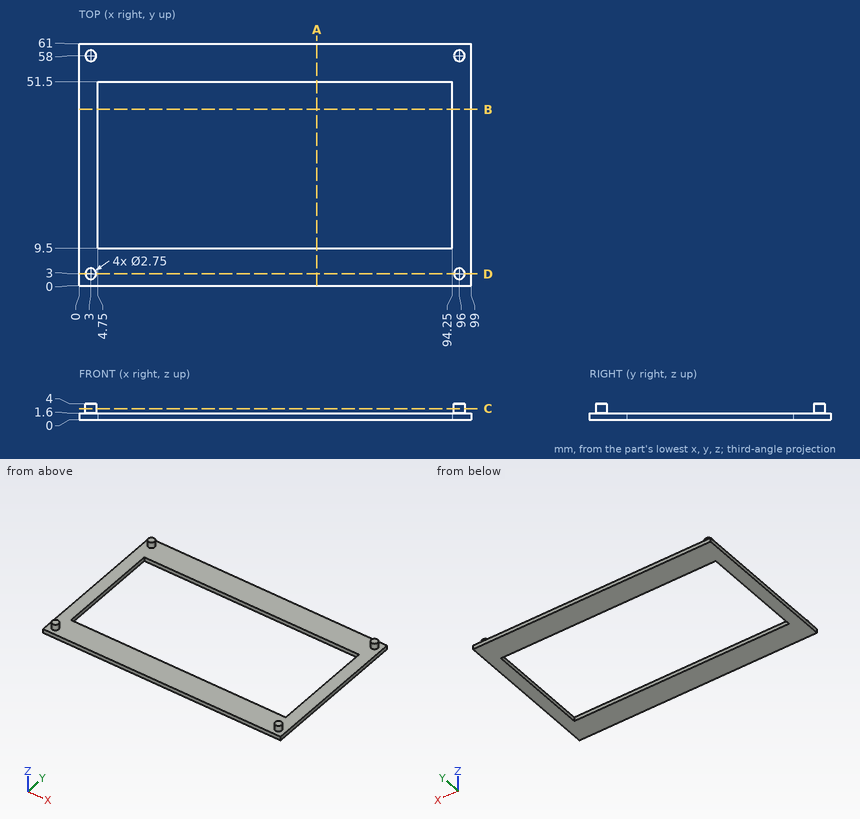
Print and shaded views of the part. All mm, measured from the part's lowest x, y and z. Round coordinates to 2 decimals unless told otherwise and drop trailing zeros. Write each loop counter-clockwise with the first axis right and the second up, starting at its lowest first coordinate (ties: lowest second). Pieces come first, ordered by that corner, then holes. Notation, with made-up numbers: (67.25, 14) -> (116.25, 14) arc R25 cw to (116.25, 33) -> close; hole circle Ø11 at (53.25, 27). An arc over 180 degrees is marked (long way). Return JSON: item names as keys, results as strings. Group by question number.
Q1. Saw through at C-C on z = 2.75. Write the cut outline in (x, y) (3 decimals), plus the area to 3 significant figures.
Q2. Saw through at A-A on x = 60. Write the cut outline in (y, z), plus the area to 3 significant figures.
Q3. Saw through at D-D on y = 3. Write the cut outline in (x, z) (3 decimals), plus the area to 3 significant figures.
Q4. Probe L1, parallel to Y at x = 53.5, z = 0.9; L2, parallel to X at y = 3, z = 3.15 (3 decimals); L3, parallel to X at y = 40.5, z = 1.1. List the from-to ranges inside material, lowest first. Write a range as [from, to].
Q5. Saw through at B-B on y = 44.5. Write the cut outline in (x, z).
Q6. Pin check, flat tip, straight feed: pin 1 (1.5 mm diameter, centred on x = 79.5, z = 2.5, fed in from +Y). Stop position of the tip, or through.
Answer:
{
 "1": {"outline": "circle Ø2.75 at (3, 3); circle Ø2.75 at (3, 58); circle Ø2.75 at (96, 3); circle Ø2.75 at (96, 58)", "area": "23.8 mm2"},
 "2": {"outline": "(0, 0) -> (9.5, 0) -> (9.5, 1.6) -> (0, 1.6) -> close; (51.5, 0) -> (61, 0) -> (61, 1.6) -> (51.5, 1.6) -> close", "area": "30.4 mm2"},
 "3": {"outline": "(0, 0) -> (99, 0) -> (99, 1.6) -> (97.375, 1.6) -> (97.375, 4) -> (94.625, 4) -> (94.625, 1.6) -> (4.375, 1.6) -> (4.375, 4) -> (1.625, 4) -> (1.625, 1.6) -> (0, 1.6) -> close", "area": "172 mm2"},
 "4": {"L1": "[0, 9.5], [51.5, 61]", "L2": "[1.625, 4.375], [94.625, 97.375]", "L3": "[0, 4.75], [94.25, 99]"},
 "5": {"outline": "(0, 0) -> (4.75, 0) -> (4.75, 1.6) -> (0, 1.6) -> close; (94.25, 0) -> (99, 0) -> (99, 1.6) -> (94.25, 1.6) -> close"},
 "6": {"pin 1": "through"}
}
